from build123d import *

# Parameters (mm, degrees)
SKETCH2_W             = 18.415
SKETCH2_H             = 1.016
BOSS_EXTRUDE1_DEPTH   = 6.35
CHAMFER1_SIZE         = 1.27
LPATTERN2_COUNT       = 7
LPATTERN2_PITCH       = 15.24
SKETCH3_W             = 20.32
SKETCH3_H             = 100.33
SKETCH3_W_2           = 16.51
SKETCH3_H_2           = 10.16
BOSS_EXTRUDE2_DEPTH   = 3.175
FILLET1_R             = 0.762
F_0_CLEARANCE_HOLE1_D = 1.8542
FILLET2_R             = 0.508
CUT_EXTRUDE1_DEPTH    = 1.5875
LPATTERN3_COUNT       = 6
LPATTERN3_PITCH       = 15.24


with BuildPart() as part:
    # Sketch2 → Boss-Extrude1 (new body)
    with BuildSketch(Plane.XY):
        with Locations((-92.71, -107.569)):
            Rectangle(SKETCH2_W, SKETCH2_H)
    extrude(amount=BOSS_EXTRUDE1_DEPTH)

    # Chamfer1
    chamfer1_edges = [part.edges().sort_by_distance(p)[0] for p in [
        (-83.5025, -107.569, 6.35),
        (-101.9175, -107.569, 6.35),
    ]]
    chamfer(chamfer1_edges, length=CHAMFER1_SIZE)


with BuildPart() as lpattern2_1:
    # LPattern2: pattern copy
    add(part.part.moved(Location(Vector(0, 1, 0) * (1 * LPATTERN2_PITCH))))


with BuildPart() as lpattern2_2:
    # LPattern2: pattern copy
    add(part.part.moved(Location(Vector(0, 1, 0) * (2 * LPATTERN2_PITCH))))


with BuildPart() as lpattern2_3:
    # LPattern2: pattern copy
    add(part.part.moved(Location(Vector(0, 1, 0) * (3 * LPATTERN2_PITCH))))


with BuildPart() as lpattern2_4:
    # LPattern2: pattern copy
    add(part.part.moved(Location(Vector(0, 1, 0) * (4 * LPATTERN2_PITCH))))


with BuildPart() as lpattern2_5:
    # LPattern2: pattern copy
    add(part.part.moved(Location(Vector(0, 1, 0) * (5 * LPATTERN2_PITCH))))


with BuildPart() as lpattern2_6:
    # LPattern2: pattern copy
    add(part.part.moved(Location(Vector(0, 1, 0) * (6 * LPATTERN2_PITCH))))


with BuildPart() as part_1:
    add(part.part)

    add(lpattern2_1.part)  # Boss-Extrude2 merges LPattern2_1

    add(lpattern2_2.part)  # Boss-Extrude2 merges LPattern2_2

    add(lpattern2_3.part)  # Boss-Extrude2 merges LPattern2_3

    add(lpattern2_4.part)  # Boss-Extrude2 merges LPattern2_4

    add(lpattern2_5.part)  # Boss-Extrude2 merges LPattern2_5

    add(lpattern2_6.part)  # Boss-Extrude2 merges LPattern2_6
    # Sketch3 → Boss-Extrude2 (add)
    with BuildSketch(Plane.XY):
        with Locations((-92.71, -61.849)):
            Rectangle(SKETCH3_W, SKETCH3_H)
        with Locations((-92.71, -99.949)):
            Rectangle(SKETCH3_W_2, SKETCH3_H_2, mode=Mode.SUBTRACT)
        with Locations((-92.71, -84.709)):
            Rectangle(SKETCH3_W_2, SKETCH3_H_2, mode=Mode.SUBTRACT)
        with Locations((-92.71, -69.469)):
            Rectangle(SKETCH3_W_2, SKETCH3_H_2, mode=Mode.SUBTRACT)
        with Locations((-92.71, -54.229)):
            Rectangle(SKETCH3_W_2, SKETCH3_H_2, mode=Mode.SUBTRACT)
        with Locations((-92.71, -38.989)):
            Rectangle(SKETCH3_W_2, SKETCH3_H_2, mode=Mode.SUBTRACT)
        with Locations((-92.71, -23.749)):
            Rectangle(SKETCH3_W_2, SKETCH3_H_2, mode=Mode.SUBTRACT)
    extrude(amount=BOSS_EXTRUDE2_DEPTH)

    # Fillet1
    fillet1_edges = [part_1.edges().sort_by_distance(p)[0] for p in [
        (-102.87, -61.849, 3.175),
        (-92.71, -112.014, 3.175),
        (-82.55, -61.849, 3.175),
        (-92.71, -11.684, 3.175),
        (-102.87, -11.684, 1.5875),
        (-102.87, -112.014, 1.5875),
        (-82.55, -112.014, 1.5875),
        (-82.55, -11.684, 1.5875),
    ]]
    fillet(fillet1_edges, radius=FILLET1_R)

    # #0 Clearance Hole1 (through all)
    with Locations(Plane.XY.offset(3.175)):
        with Locations((-97.409, -13.6525), (-88.011, -13.6525), (-97.409, -110.0455), (-88.011, -110.0455)):
            Hole(F_0_CLEARANCE_HOLE1_D / 2)

    # Fillet2
    fillet2_edges = [part_1.edges().sort_by_distance(p)[0] for p in [
        (-84.455, -94.869, 1.5875),
        (-100.965, -94.869, 1.5875),
        (-100.965, -105.029, 1.5875),
        (-84.455, -105.029, 1.5875),
        (-84.455, -89.789, 1.5875),
        (-84.455, -79.629, 1.5875),
        (-100.965, -79.629, 1.5875),
        (-100.965, -89.789, 1.5875),
        (-84.455, -74.549, 1.5875),
        (-84.455, -64.389, 1.5875),
        (-100.965, -64.389, 1.5875),
        (-100.965, -74.549, 1.5875),
        (-84.455, -59.309, 1.5875),
        (-84.455, -49.149, 1.5875),
        (-100.965, -49.149, 1.5875),
        (-100.965, -59.309, 1.5875),
        (-84.455, -44.069, 1.5875),
        (-84.455, -33.909, 1.5875),
        (-100.965, -33.909, 1.5875),
        (-100.965, -44.069, 1.5875),
        (-84.455, -28.829, 1.5875),
        (-84.455, -18.669, 1.5875),
        (-100.965, -18.669, 1.5875),
        (-100.965, -28.829, 1.5875),
    ]]
    fillet(fillet2_edges, radius=FILLET2_R)

    # Sketch9 → Cut-Extrude1 (cut)
    with BuildSketch(Plane(origin=(0, 0, 0), x_dir=(-1, 0, 0), z_dir=(0, 0, -1))):
        with BuildLine():
            Line((102.235, -105.283), (102.235, -94.615))
            ThreePointArc((102.235, -94.615), (101.93742049, -93.89657951), (101.219, -93.599))
            Line((101.219, -93.599), (84.201, -93.599))
            ThreePointArc((84.201, -93.599), (83.48257951, -93.89657951), (83.185, -94.615))
            Line((83.185, -94.615), (83.185, -105.283))
            ThreePointArc((83.185, -105.283), (83.48257951, -106.00142049), (84.201, -106.299))
            Line((84.201, -106.299), (101.219, -106.299))
            ThreePointArc((101.219, -106.299), (101.93742049, -106.00142049), (102.235, -105.283))
        make_face()
    cut_extrude1 = extrude(amount=-CUT_EXTRUDE1_DEPTH, mode=Mode.SUBTRACT)

    # LPattern3: Cut-Extrude1 ×6
    with Locations(*[(0, i * LPATTERN3_PITCH, 0) for i in range(1, LPATTERN3_COUNT)]):
        add(cut_extrude1, mode=Mode.SUBTRACT)


solid = part_1.part
Here's how the part is built. I have some questions about the finished solid (model axes, mm). A direction names the side the tool comes from. Coordinates: 2 decimals unless noted, no trailing zeros. Order: outer loops, then holes, each group sorted by start corner. A loop starts at its lowest first (then second) coordinate and runs counter-clockwise, first axis right, second up. Notation, with made-up numbers: M 86,58 L 132,58 A29 cw 132,90 Z; hole C -38.75,-32.75 d10. An arc over 180 degrees is marked long. Answer as CSV lines item,"result". Start each with the question number.
1. I want a section at C-C, the plane x = -95.5. Count the separate pieces of the cut face and the enclosed holes in it, and give its area (3 significant figures).
2. We'd pull the mould along X, two halves only. Please class faces 4 (the flat face through (-93, -59.309, 2)), 5 (the flat face through (-82.55, -63, 1)), 6 (the flat face through (-93, -16.637, 5)): released by +X, released by -X, zero draft, split by the parting line, or undercut.
3. I need wall thicknesses on line 1 (X direction, y = -52, z = 1) (3 decimals); line 2 (Z direction, x = -83.75, y = -84) (1 decimal); line 3 (X direction, y = -100.5, z = 2) (3 decimals). Which ranges of each line are inside material? Lowest first, please. Write a range as [from, to].
4. For pin 1 (3 mm diameter, centred on x = -89, y = -58, fed in from +Z) (3 decimals); pin 2 (1.6 mm diameter, centred on x = -91.5, z = 5.5, fed in from +Y); pin 3 (6.5 mm diameter, centred on x = -89, y = -102, fed in from -Z), each with a flat end and sliding along its axis, tell me the tip position at first contact or that it passes through.
5. On a 3-axis mill with a long thin cutter (end or side, diameter ignored), from which of +Z, -Z, +X, -X, +Y, -Y can I reach the whole of each face in a straight line? I mean faces 1 (the flat face through (-93, -30.861, 5)), 2 (the flat face through (-93, -106.299, 1)), 3 (the flat face through (-100.965, -70, 2)). Say none if no direction works.
6. I want a section at A-A, the plane z = 4. Write out the boundary of the cut face in (x, y), and give its area (3 significant figures).
Recorded:
1,separate pieces,"7"
1,enclosed holes,"0"
1,area,"123 mm2"
2,face 4,"undercut"
2,face 5,"released by +X"
2,face 6,"zero draft"
3,line 1,"x = [-102.87, -102.235], [-83.185, -82.55]"
3,line 2,"z = [1.6, 3.2]"
3,line 3,"x = [-102.87, -100.965], [-84.455, -82.55]"
4,pin 1,"stops at z = 3.175"
4,pin 2,"stops at y = -15.62"
4,pin 3,"stops at z = 1.59"
5,face 1,"+Z, +X, -X"
5,face 2,"-Z"
5,face 3,"+Z, -Z"
6,outline,"M -101.92,-108.08 L -83.5,-108.08 L -83.5,-107.06 L -101.92,-107.06 Z; M -101.92,-92.84 L -83.5,-92.84 L -83.5,-91.82 L -101.92,-91.82 Z; M -101.92,-77.6 L -83.5,-77.6 L -83.5,-76.58 L -101.92,-76.58 Z; M -101.92,-62.36 L -83.5,-62.36 L -83.5,-61.34 L -101.92,-61.34 Z; M -101.92,-47.12 L -83.5,-47.12 L -83.5,-46.1 L -101.92,-46.1 Z; M -101.92,-31.88 L -83.5,-31.88 L -83.5,-30.86 L -101.92,-30.86 Z; M -101.92,-16.64 L -83.5,-16.64 L -83.5,-15.62 L -101.92,-15.62 Z"
6,area,"131 mm2"
